from build123d import *

# Parameters (mm, degrees)
F0_W     = 27
F0_H     = 55.25
F1_DEPTH = 15
F2_R     = 4
F3_T     = -1.2


with BuildPart() as f1:
    # F0 (on Front) → F1 (new body)
    with BuildSketch(Plane.XZ):
        Rectangle(F0_W, F0_H)
    extrude(amount=F1_DEPTH)

    # F2
    f2_edges = [f1.edges().sort_by_distance(p)[0] for p in [
        (13.5, -15, 0),
        (-13.5, -15, 0),
    ]]
    fillet(f2_edges, radius=F2_R)

    # F3
    f3_openings = [f1.faces().sort_by_distance(p)[0] for p in [
        (0, 0, 0),
    ]]
    offset(amount=F3_T, openings=f3_openings)


solid = f1.part
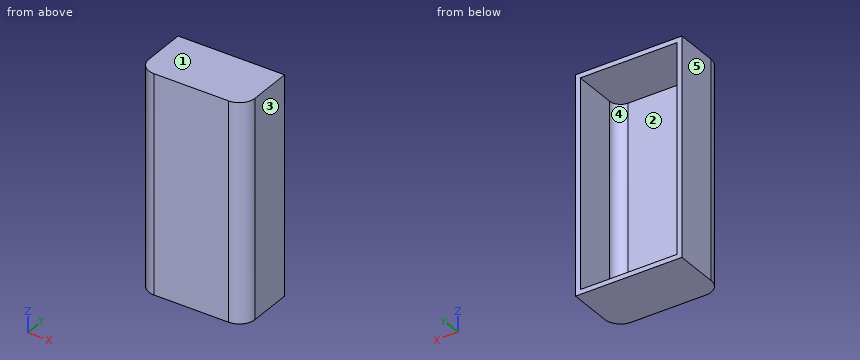
Geometry check sheet. Reference: the model listing, model coordinates, mm. Face numbers are marked on the shaded views. A direction names the side the tool comes from. Round coordinates to 2 decimals unless told otherwise and drop trailing zeros. Order: outer loops, then holes, each group sorted by start corner. A loop starts at its lowest first (then second) coordinate and runs counter-clockwise, first axis right, second up. Notation, with made-up numbers: (82, 63.25) - (87, 63.25) arc R5 cw to (87, 71.25) - close; hole circle Ø8 at (-22, -39). An arc over 180 degrees is marked (long way). One line per question, with ' | ' between items. Start each with the question number.
(1) Sectioned sample at B-B on y = -6. Record the cut outline in (x, z) (3 decimals), and give its area (3 significant figures).
(2) Sectioned sample at D-D on y = -13. Record the cut outline in (x, z) (3 decimals), and give its area (3 significant figures).
(3) Thickness scan on L1, parallel to Z at x = -4.25, y = -6.5 (3 decimals); L2, parallel to X at y = -6, z = 5.5; L3, parallel to Y at x = 3, z = 21. Record the ranges inside material, lowest first. Write a range as [from, to].
(4) Release check for a two-part mould opening along Z. For the marked faces 1, 2 and 3 record: released by +Z, released by -Z, zero draft, split by the parting line, or undercut.
(5) Access from +Z, -Z, +X, -X, +Y, -Y to the whole of each face (thin tool, end or side, straight path). Record for the marked faces 4 and 5.
(6) Depth check by flat-ended pin: pin 1 Ø15 at (x, z) = (-1, 3) entering from +Y; pin 2 Ø1 at (y, z) = (-12, -18) entering from +X; pin 3 Ø3 at (x, z) = (9, 20.5) entering from +Y. Enter the tip coordinate at first touch or a pass-through.
(7) Sectioned sample at A-A on z = 23.5. Record the cut outline in (x, y), and give its area (3 significant figures).
(8) Sectioned sample at C-C on x = 1.5. Record the cut outline in (y, z) (3 decimals), and give its area (3 significant figures).
Conclusion:
1) outline: (-13.5, -27.625) - (13.5, -27.625) - (13.5, 27.625) - (-13.5, 27.625) - close; hole (-12.3, -26.425) - (12.3, -26.425) - (12.3, 26.425) - (-12.3, 26.425) - close | area: 192 mm2
2) outline: (-12.964, -27.625) - (12.964, -27.625) - (12.964, 27.625) - (-12.964, 27.625) - close; hole (-11.46, -26.425) - (11.46, -26.425) - (11.46, 26.425) - (-11.46, 26.425) - close | area: 221 mm2
3) L1: z = [-27.625, -26.425], [26.425, 27.625] | L2: x = [-13.5, -12.3], [12.3, 13.5] | L3: y = [-15, -13.8]
4) face 1: released by +Z | face 2: undercut | face 3: zero draft
5) face 4: +Y | face 5: +Z, -Z, -X, +Y, -Y
6) pin 1: stops at y = -13.8 | pin 2: stops at x = 13.47 | pin 3: stops at y = -13.62
7) outline: (-13.5, -11) arc R4 ccw to (-9.5, -15) - (9.5, -15) arc R4 ccw to (13.5, -11) - (13.5, 0) - (12.3, 0) - (12.3, -11) arc R2.8 cw to (9.5, -13.8) - (-9.5, -13.8) arc R2.8 cw to (-12.3, -11) - (-12.3, 0) - (-13.5, 0) - close | area: 62.0 mm2
8) outline: (-15, -27.625) - (0, -27.625) - (0, -26.425) - (-13.8, -26.425) - (-13.8, 26.425) - (0, 26.425) - (0, 27.625) - (-15, 27.625) - close | area: 99.4 mm2
